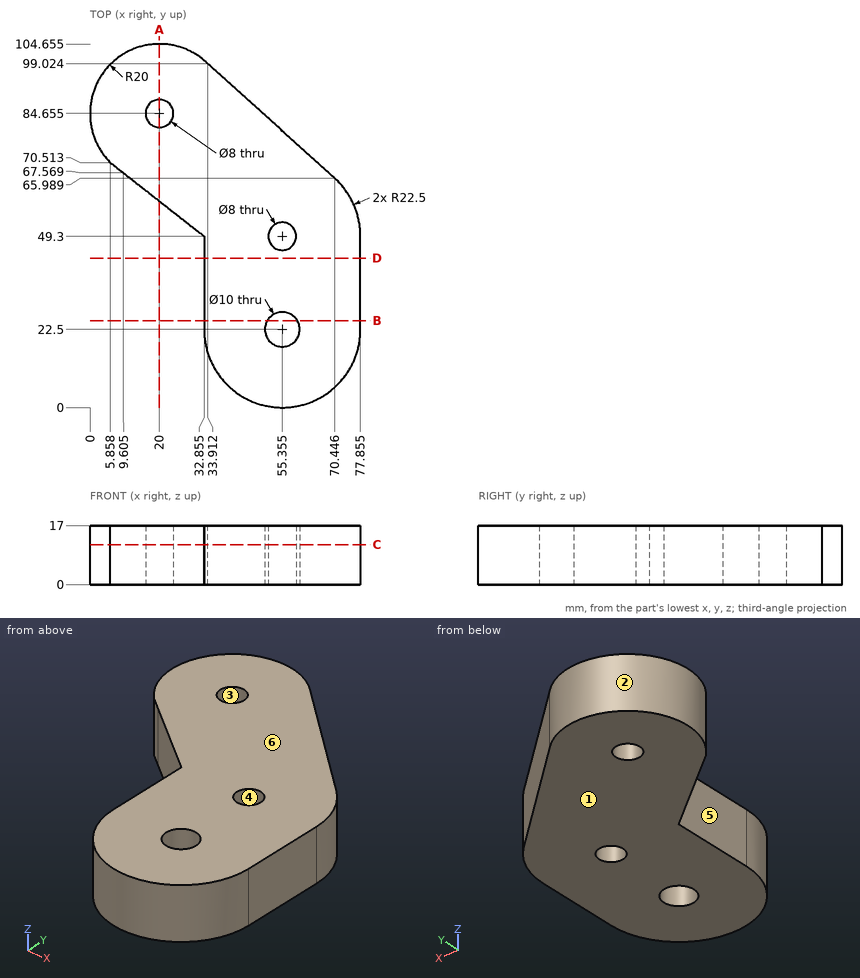
Input: dimensioned drawing with shaded views. Units: mm. Origin: part minimum x, y, z. A direction names the side the tool comes from. Give positions to 0.01 mm unless a question says otherwise; leave off trailing zeros. Loops run counter-clockwise (first coordinate to the right, second up) from the corner with the lowest first, then second, coordinate; pieces in that order, holes last. Notation, with made-up numbers: M 16.5,0 L 62.5,0 A17 cw 62.5,11 Z; hole C 88,72.25 d10. An arc over 180 degrees is marked long. Put each result on its own line as item: value. Start each with the question number.
1) Cut plane A-A (x = 20). Output: boundary loops of the cut face in (y, z) (1 decimal).
2) Cut plane D-D (y = 43). Output: boundary loops of the cut face in (x, z) (1 decimal), then the cut area to 3 significant figures.
3) Contact query for flat-ended pins moving along their axis: pin 1 (9 mm diameter, centred on x = 55.36, y = 49.3, fed in from +Z); pin 2 (3 mm diameter, centred on x = 39.5, z = 7, fed in from +Y); pin 3 (6 mm diameter, centred on y = 33.5, z = 12.5, fed in from -X) (1 decimal); pin 4 (2 mm diameter, centred on y = 92.5, z = 2, fed in from +X). Output: stop coordinate, or through.
4) Cut plane C-C (z = 11.5). Output: boundary loops of the cut face in (x, y) (1 decimal).
5) Ray query, line 1 along X through (y, z) = (84, 1.5) (1 decimal); line 2 along Y through (x, z) = (20, 7.25) (1 decimal); line 3 along Y through (x, z) = (23, 10.25) (1 decimal). Return the intervals inside material, ascending.
6) Cut plane B-B (y = 25). Output: boundary loops of the cut face in (x, z) (1 decimal), then the cut area to 3 significant figures.
7) Access query for the marked faces 5 and 6. Directions: +Z, -Z, +X, -X, +Y, -Y. A direction counts if a zero-diameter tool reaches every point of the face in a straight line with its end or side. Return the directions, or none.
8) Pull-direction query (Y, two-part tool) for the marked faces 1, 2, 3 and 4; classes: pulls with the +Y half, pulls with the -Y half, needs draft (parallel to the pull), parting line crosses it, or undercut.
Verdict:
1. outline: M 59.4,0 L 80.7,0 L 80.7,17 L 59.4,17 Z; M 88.7,0 L 104.7,0 L 104.7,17 L 88.7,17 Z
2. outline: M 32.9,0 L 77.9,0 L 77.9,17 L 32.9,17 Z
2. area: 765 mm2
3. pin 1: z = 17
3. pin 2: y = 95.33
3. pin 3: x = 32.9
3. pin 4: x = 42.23
4. outline: M 5.9,70.5 L 32.9,49.3 L 32.9,22.5 A22.5 ccw 77.9,22.5 L 77.9,49.3 A22.5 ccw 70.4,66 L 33.9,99 A20 ccw Z; hole C 20,84.7 d8; hole C 55.4,22.5 d10; hole C 55.4,49.3 d8
5. line 1: 0 to 16.1, 23.9 to 50.5
5. line 2: 59.4 to 80.7, 88.7 to 104.7
5. line 3: 57 to 82, 87.3 to 104.4
6. outline: M 32.9,0 L 51,0 L 51,17 L 32.9,17 Z; M 59.7,0 L 77.9,0 L 77.9,17 L 59.7,17 Z
6. area: 618 mm2
7. face 5: +Z, -Z, -X, -Y
7. face 6: +Z, +X, -X, +Y, -Y
8. face 1: needs draft
8. face 2: parting line crosses it
8. face 3: undercut
8. face 4: undercut
